Autodesk Fusion 360 part; units mm, degrees
sketch "Sketch1" plane through (0, 0, 0) normal (0, 0, 1) x (1, 0, 0)
  arc A0 (2.4187, -2.2) -> (2.4187, 2.2) centre (1.4436, 0) ccw
  line L0 (-2.4187, 2.2) -> (2.4187, 2.2)
  arc A1 (-2.4187, 2.2) -> (-2.4187, -2.2) centre (-1.4436, 0) ccw
  line L1 (2.4187, -2.2) -> (-2.4187, -2.2)
  line L2 (6.85, -2.55) -> (-6.85, -2.55)
  line L3 (-6.85, 2.55) -> (-6.85, -2.55)
  line L4 (6.85, 2.55) -> (-6.85, 2.55)
  line L5 (6.85, 2.55) -> (6.85, -2.55)
  arc A2 (2.45, -2.35) -> (2.45, 2.35) centre (1.4436, 0) ccw
  line L6 (-2.45, 2.35) -> (2.45, 2.35)
  arc A3 (-2.45, 2.35) -> (-2.45, -2.35) centre (-1.4436, 0) ccw
  line L7 (2.45, -2.35) -> (-2.45, -2.35)
  dimension "d33" = 0.15
extrude "Extrude3" add sketch "Sketch1" against normal blind 0.4 contours A0 L0 A1 L1 | L2 L3 L4 L5 | A2 L6 A3 L7
extrude "Extrude4" add sketch "Sketch1" along normal blind 4.4 contours A0 L0 A1 L1 | A2 L6 A3 L7
extrude "Extrude7" cut 1 faces at (6.85, 0.85, -0.1333) along direction (-1, 0, 0) blind 1
extrude "Extrude8" cut 1 faces at (-6.85, 0.85, -0.1333) along direction (1, 0, 0) blind 1
fillet "Fillet3" radius 1 4 edges at (-4, 0, 4.4) (0, -2.35, 4.4) (0, 2.35, 4.4) (4, 0, 4.4)
extrude "Extrude9" cut 1 faces at (-1.95, -2.55, -0.2667) along direction (0, 1, 0) up to surface (0.2 mm away)
extrude "Extrude10" cut 1 faces at (-1.95, 2.55, -0.2667) along direction (0, -1, 0) up to surface (0.2 mm away)
sketch "Sketch2" plane through (0, -2.35, 0) normal (0, -1, 0) x (1, 0, 0)
  line L0 (2.45, 3.4) -> (-2.45, 3.4)
  line L1 (-2.45, 3.4) -> (-2.45, 0)
  line L2 (-2.45, 0) -> (-5.85, 0)
  line L3 (-5.85, 0) -> (-5.85, -0.4)
  line L4 (-5.85, -0.4) -> (5.85, -0.4)
  line L5 (5.85, -0.4) -> (5.85, 0)
  line L6 (5.85, 0) -> (2.45, 0)
  line L7 (2.45, 0) -> (2.45, 3.4)
  line L8 (-2.45, 0) -> (2.45, 0)
sketch "Sketch3" plane through (0, 2.35, 0) normal (0, 1, 0) x (-1, 0, 0)
  line L0 (2.45, 3.4) -> (-2.45, 3.4)
  line L1 (-2.45, 3.4) -> (-2.45, 0)
  line L2 (-2.45, 0) -> (-5.85, 0)
  line L3 (-5.85, 0) -> (-5.85, -0.4)
  line L4 (-5.85, -0.4) -> (5.85, -0.4)
  line L5 (5.85, -0.4) -> (5.85, 0)
  line L6 (5.85, 0) -> (2.45, 0)
  line L7 (2.45, 0) -> (2.45, 3.4)
  line L8 (-2.45, 0) -> (2.45, 0)
chamfer "Chamfer2" distance 0.4 angle 45 2 edges at (0, 2.35, -0.4) (0, -2.35, -0.4)
The model under review builds one solid part; all positions refer to its coordinate system, in mm. A direction names the side the tool comes from. Round coordinates to 2 decimals unless told otherwise and drop trailing zeros. Write each loop counter-clockwise with the first axis right and the second up, starting at its lowest first coordinate (ties: lowest second). Pieces come first, ordered by that corner, then holes.
(1) We need section B-B on y = 0. Give the boundary of the cut face in (x, z).
(2) Insertion check: pin 1 (2 mm diameter, centred on x = -4, z = 2, fed in from +Y). The pin has a flat end and moves straight along its axis. Give the tip position at first contact, or say it passes through.
(3) We need section A-A on x = -0.5. Give the boundary of the cut face in (y, z), and give its area (3 significant figures).
(4) Machinability: for faces 1 (the cylindrical face through (-4, 0, 2)), 2 (the cylindrical face through (4, 0, 2)), 3 (the flat face through (0, 0, -0.4)), which of the approach directions +Z, -Z, +X, -X, +Y, -Y give a long, thin tool a straight path to every point of the face, cutting with its end or side? Answer none if there is none.
(5) We need section C-C on z = 0.9. Give the boundary of the cut face in (x, y), and give its area (3 significant figures).
(6) Wall thickness on L1, parallel to Z at x = 5.25, y = 1.1; L2, parallel to X at y = -0.25, z = 2.7; L3, parallel to Z at x = 1.5, y = -1.8: over which ranges is each line inside the solid? List them lowest first.
(7) We need section D-D on z = 4.1. Give the boundary of the cut face in (x, y), and give its area (3 significant figures).
Findings below:
1. outline: (-5.85, -0.4) - (5.85, -0.4) - (5.85, 0) - (4, 0) - (4, 3.4) arc R1 ccw to (3, 4.4) - (-3, 4.4) arc R1 ccw to (-4, 3.4) - (-4, 0) - (-5.85, 0) - close
2. pin 1: stops at y = 2.03
3. outline: (-2.35, 0) - (-1.95, -0.4) - (1.95, -0.4) - (2.35, 0) - (2.35, 3.4) arc R1 ccw to (1.35, 4.4) - (-1.35, 4.4) arc R1 ccw to (-2.35, 3.4) - close
3. area: 22.0 mm2
4. face 1: +Z, -X
4. face 2: +Z, +X
4. face 3: -Z, +X, -X, +Y, -Y
5. outline: (-2.45, -2.35) - (2.45, -2.35) arc R2.56 ccw to (2.45, 2.35) - (-2.45, 2.35) arc R2.56 ccw to start
5. area: 33.5 mm2
6. L1: z = -0.4 to 0
6. L2: x = -3.99 to 3.99
6. L3: z = -0.4 to 4.29
7. outline: (-2.39, -2.06) - (2.39, -2.06) arc R2.27 ccw to (2.39, 2.06) - (-2.39, 2.06) arc R2.27 ccw to start
7. area: 27.6 mm2
